Could you check a few things on this model? Use its own coordinates, in mm. A direction names the side the tool comes from. Give positions to 0.01 mm unless a question says otherwise; leave off trailing zeros. Loops run counter-clockwise (first coordinate to the right, second up) from the corner with the lowest first, then second, coordinate; pieces in that order, holes last.
1. Imagine slicing it at B-B (x = -0.5). List the corners of the cut face in (y, z) for me, plus the area to 3 significant figures.
2. Imagine slicing it at D-D (y = 4.5). List the corners of the cut face in (x, z) for me (3 decimals).
3. Imagine slicing it at A-A (y = -10). List the corners of the cut face in (x, z) for me (3 decimals).
4. Thinking about a two-plate mould opening in Z: for faces 1 (the flat face through (0, 0, -10)), 2 (the flat face through (0, 0, 5)), 3 (the cylindrical face through (0.04, -6.35, -28.4)), 4 (the flat face through (0, 7.62, -9)), which applies, +Z half, -Z half, draft (parallel to the pull), parting line (faces both ways), or undercut?
5. I need wall thicknesses on line 1 along Z through (x, y) = (20.5, 14.5); line 2 along Z through (x, y) = (-2, -0.5); line 3 along X through (y, z) = (5, -18) (3 decimals). Which ranges of each line are inside material? Lowest first, please.
6. For P1, Ø12, axis at x = 0.5, y = -4.5, coming from the -Z side; P2, Ø2, axis at x = 7, y = -14, coming from the -Z side; P3, Ø15, axis at x = 1, y = 10.5, coming from the -Z side; P4, Ø2, axis at x = -6, z = -15.5, coming from the -Y side, each with a flat end and sliding along its axis, tell me the tip position at first contact or that it passes through.
7. Imagine slicing it at C-C (z = -11). List the corners of the cut face in (x, y) for me (3 decimals).
8. For faces 5 (the flat face through (-3.175, 1, -17)), 6 (the flat face through (3.175, 0.2, -17)), 7 (the flat face through (25.4, 0, 2)), which set-ups out of +Z, -Z, +X, -X, +Y, -Y let a thin tool reach every point of the face, with its end or its side?
```python
from build123d import *

# Parameters (mm, degrees)
F0_W     = 50.8
F0_H     = 50.8
F1_DEPTH = 5
F2_W     = 7.62
F2_H     = 19.05
F3_DEPTH = 3.175
F4_DEPTH = 3.175


with BuildPart() as f1:
    # F0 (on Top) → F1 (new body)
    with BuildSketch(Plane.XY):
        Rectangle(F0_W, F0_H)
    extrude(amount=F1_DEPTH)

    # F2 (on Right) → F3 (join)
    with BuildSketch(Plane.YZ):
        with Locations((3.81, -9.525)):
            Rectangle(F2_W, F2_H)
        with BuildLine():
            Line((7.62, -19.05), (0, -19.05))
            ThreePointArc((0, -19.05), (-6.23626, -28.293401), (-15.736038, -34.131691))
            ThreePointArc((-15.736038, -34.131691), (-1.531188, -30.503985), (7.62, -19.05))
        make_face()
    extrude(amount=F3_DEPTH)

    # F3_face (on face) → F4 (join)
    with BuildSketch(Plane(origin=(0, 1.478785, -16.812589), x_dir=(0, 1, 0), z_dir=(-1, 0, 0))):
        with BuildLine():
            Line((-1.478785, -16.812589), (6.141215, -16.812589))
            Line((6.141215, -16.812589), (6.141215, 2.237411))
            ThreePointArc((6.141215, 2.237411), (-3.009973, 13.691396), (-17.214823, 17.319102))
            ThreePointArc((-17.214823, 17.319102), (-7.715045, 11.480812), (-1.478785, 2.237411))
            Line((-1.478785, 2.237411), (-1.478785, -16.812589))
        make_face()
    extrude(amount=F4_DEPTH)


solid = f1.part
```
Derived:
1. outline: (-25.4, 0) - (0, 0) - (0, -19.05) arc R26.36 cw to (-15.74, -34.13) arc R23.07 ccw to (7.62, -19.05) - (7.62, 0) - (25.4, 0) - (25.4, 5) - (-25.4, 5) - close
1. area: 510 mm2
2. outline: (-25.4, 0) - (-3.175, 0) - (-3.175, -24.845) - (3.175, -24.845) - (3.175, 0) - (25.4, 0) - (25.4, 5) - (-25.4, 5) - close
3. outline: (-25.4, 0) - (25.4, 0) - (25.4, 5) - (-25.4, 5) - close; (-3.175, -33.836) - (3.175, -33.836) - (3.175, -31.292) - (-3.175, -31.292) - close
4. face 1: undercut
4. face 2: +Z half
4. face 3: undercut
4. face 4: draft
5. line 1: z = 0 to 5
5. line 2: z = -29.8 to -20.22, 0 to 5
5. line 3: x = -3.175 to 3.175
6. P1: stops at z = -33.92
6. P2: stops at z = 0
6. P3: stops at z = -26.67
6. P4: passes through
7. outline: (-3.175, 0) - (3.175, 0) - (3.175, 7.62) - (-3.175, 7.62) - close
8. face 5: -Z, -X, +Y, -Y
8. face 6: -Z, +X, +Y, -Y
8. face 7: +Z, -Z, +X, +Y, -Y
